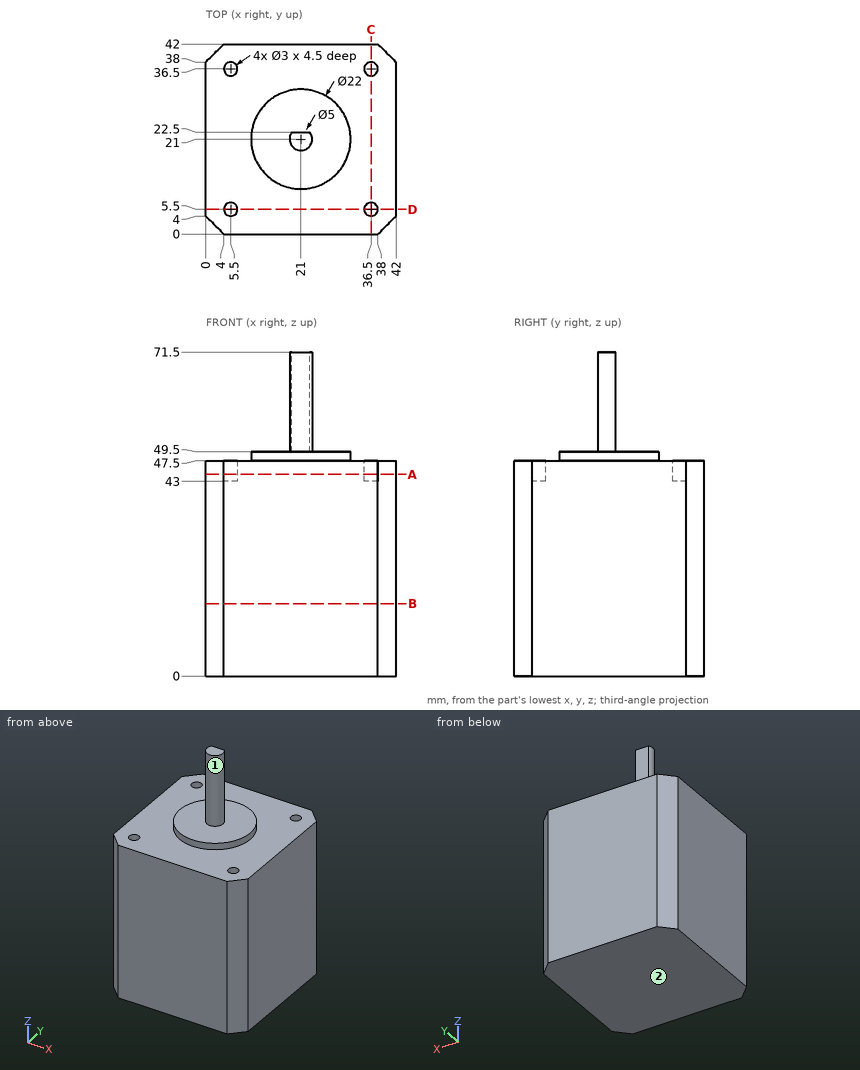
Input: dimensioned drawing with shaded views. Units: mm. Origin: part minimum x, y, z. A direction names the side the tool comes from. Give positions to 0.01 mm unless a question says otherwise; leave off trailing zeros. Order: outer loops, then holes, each group sorted by start corner. A loop starts at its lowest first (then second) coordinate and runs counter-clockwise, first axis right, second up. Notation, with made-up numbers: (16, 84.25) -> (37, 84.25) arc R23 cw to (37, 93.25) -> close; hole circle Ø6 at (-34, -13). An arc over 180 degrees is marked (long way). Use one line per item in the form item = value.
1) Section A-A, the plane z = 44.5. Return loops of the section in (x, y), and give its area (3 significant figures).
Response values:
outline = (0, 4) -> (4, 0) -> (38, 0) -> (42, 4) -> (42, 38) -> (38, 42) -> (4, 42) -> (0, 38) -> close; hole circle Ø3 at (5.5, 5.5); hole circle Ø3 at (5.5, 36.5); hole circle Ø3 at (36.5, 5.5); hole circle Ø3 at (36.5, 36.5)
area = 1,700 mm^2
2) First-contact query: pin 1 Ø10 at (y, z) = (24, 59) entering from -X; pin 2 Ø1.5 at (x, y) = (5, 36) entering from +Z; pin 3 Ø1.2 at (x, z) = (21.5, 61.5) entering from +Y. Flat tips, straight axial feed; report the tip coordinate or a pass-through.
Response values:
pin_1 = 18.5
pin_2 = 43
pin_3 = 22.5
3) Section C-C, the plane x = 36.5. Return loops of the section in (y, z), and give its area (3 significant figures).
Response values:
outline = (0, 0) -> (42, 0) -> (42, 47.5) -> (38, 47.5) -> (38, 43) -> (35, 43) -> (35, 47.5) -> (7, 47.5) -> (7, 43) -> (4, 43) -> (4, 47.5) -> (0, 47.5) -> close
area = 1,970 mm^2
4) Reachability of the marked faces 1 and 2 from +Z, -Z, +X, -X, +Y, -Y: full face, straight path, thin tool, end or side. Return the list, or none.
Response values:
face_1 = +Z
face_2 = -Z, +X, -X, +Y, -Y
5) Section B-B, the plane z = 16. Return loops of the section in (x, y).
Response values:
outline = (0, 4) -> (4, 0) -> (38, 0) -> (42, 4) -> (42, 38) -> (38, 42) -> (4, 42) -> (0, 38) -> close
6) Line query: probe 1 along Y at (x, z) = (5.5, 45.9); probe 2 along Y at (x, z) = (5, 45); probe 3 along Z at (x, y) = (20, 7). Output: solid intervals per line, ascending.
Response values:
probe_1 = 0 to 4, 7 to 35, 38 to 42
probe_2 = 0 to 4.09, 6.91 to 35.09, 37.91 to 42
probe_3 = 0 to 47.5
